Geometry check sheet. Reference: the model listing, model coordinates, mm. A direction names the side the tool comes from. Round coordinates to 2 decimals unless told otherwise and drop trailing zeros. Order: outer loops, then holes, each group sorted by start corner. A loop starts at its lowest first (then second) coordinate and runs counter-clockwise, first axis right, second up. Notation, with made-up numbers: M 13.25,32 L 37.25,32 A28 ccw 37.25,58 Z; hole C -2.5,-11.75 d11. An arc over 180 degrees is marked long. Return JSON: item names as keys, results as strings. Group by question number.
```python
from build123d import *

# Parameters (mm, degrees)
F1_DEPTH = 6.35


with BuildPart() as f1:
    # F0 (on Top) → F1 (new body)
    with BuildSketch(Plane.XY):
        with BuildLine():
            Line((1.27, 15.24), (-1.27, 15.24))
            ThreePointArc((-1.27, 15.24), (-2.121422, 13.939986), (-2.54, 12.443408))
            ThreePointArc((-2.54, 12.443408), (-3.578003, 12.185561), (-4.59063, 11.841289))
            ThreePointArc((-4.59063, 11.841289), (-5.751872, 12.87399), (-7.170974, 13.507318))
            Line((-7.170974, 13.507318), (-9.307758, 12.13409))
            ThreePointArc((-9.307758, 12.13409), (-9.321179, 10.580136), (-8.864198, 9.094833))
            ThreePointArc((-8.864198, 9.094833), (-9.59802, 8.316731), (-10.263768, 7.479644))
            ThreePointArc((-10.263768, 7.479644), (-11.798987, 7.720592), (-13.335215, 7.486157))
            Line((-13.335215, 7.486157), (-14.390369, 5.175692))
            ThreePointArc((-14.390369, 5.175692), (-13.561528, 3.861167), (-12.374076, 2.858713))
            ThreePointArc((-12.374076, 2.858713), (-12.570732, 1.807398), (-12.678232, 0.743265))
            ThreePointArc((-12.678232, 0.743265), (-14.100007, 0.115962), (-15.265619, -0.911805))
            Line((-15.265619, -0.911805), (-14.904139, -3.425951))
            ThreePointArc((-14.904139, -3.425951), (-13.496187, -4.083695), (-11.955272, -4.285028))
            ThreePointArc((-11.955272, -4.285028), (-11.552326, -5.275771), (-11.067446, -6.229095))
            ThreePointArc((-11.067446, -6.229095), (-11.924374, -7.525486), (-12.349297, -9.020276))
            Line((-12.349297, -9.020276), (-10.68595, -10.93988))
            ThreePointArc((-10.68595, -10.93988), (-9.145903, -10.732013), (-7.740754, -10.068303))
            ThreePointArc((-7.740754, -10.068303), (-6.866138, -10.68392), (-5.942825, -11.223762))
            ThreePointArc((-5.942825, -11.223762), (-5.962837, -12.777645), (-5.51216, -14.264873))
            Line((-5.51216, -14.264873), (-3.075048, -14.980473))
            ThreePointArc((-3.075048, -14.980473), (-1.891859, -13.972992), (-1.068601, -12.654963))
            ThreePointArc((-1.068601, -12.654963), (0, -12.7), (1.068601, -12.654963))
            ThreePointArc((1.068601, -12.654963), (1.891859, -13.972992), (3.075048, -14.980473))
            Line((3.075048, -14.980473), (5.51216, -14.264873))
            ThreePointArc((5.51216, -14.264873), (5.962837, -12.777645), (5.942825, -11.223762))
            ThreePointArc((5.942825, -11.223762), (6.866138, -10.68392), (7.740754, -10.068303))
            ThreePointArc((7.740754, -10.068303), (9.145903, -10.732013), (10.68595, -10.93988))
            Line((10.68595, -10.93988), (12.349297, -9.020276))
            ThreePointArc((12.349297, -9.020276), (11.924374, -7.525486), (11.067446, -6.229095))
            ThreePointArc((11.067446, -6.229095), (11.552326, -5.275771), (11.955272, -4.285028))
            ThreePointArc((11.955272, -4.285028), (13.496187, -4.083695), (14.904139, -3.425951))
            Line((14.904139, -3.425951), (15.265619, -0.911805))
            ThreePointArc((15.265619, -0.911805), (14.100007, 0.115962), (12.678232, 0.743265))
            ThreePointArc((12.678232, 0.743265), (12.570732, 1.807398), (12.374076, 2.858713))
            ThreePointArc((12.374076, 2.858713), (13.561528, 3.861167), (14.390369, 5.175692))
            Line((14.390369, 5.175692), (13.335215, 7.486157))
            ThreePointArc((13.335215, 7.486157), (11.798987, 7.720592), (10.263768, 7.479644))
            ThreePointArc((10.263768, 7.479644), (9.59802, 8.316731), (8.864198, 9.094833))
            ThreePointArc((8.864198, 9.094833), (9.321179, 10.580136), (9.307758, 12.13409))
            Line((9.307758, 12.13409), (7.170974, 13.507318))
            ThreePointArc((7.170974, 13.507318), (5.751872, 12.87399), (4.59063, 11.841289))
            ThreePointArc((4.59063, 11.841289), (3.578003, 12.185561), (2.54, 12.443408))
            ThreePointArc((2.54, 12.443408), (2.121422, 13.939986), (1.27, 15.24))
        make_face()
        with BuildLine():
            ThreePointArc((-1.717218, -6.1134), (0, 6.35), (1.717218, -6.1134))
            ThreePointArc((1.717218, -6.1134), (1.623593, -6.177189), (1.5875, -6.284575))
            Line((1.5875, -6.284575), (1.5875, -9.3472))
            ThreePointArc((1.5875, -9.3472), (1.535424, -9.472924), (1.4097, -9.525))
            Line((1.4097, -9.525), (-1.4097, -9.525))
            ThreePointArc((-1.4097, -9.525), (-1.535424, -9.472924), (-1.5875, -9.3472))
            Line((-1.5875, -9.3472), (-1.5875, -6.284575))
            ThreePointArc((-1.5875, -6.284575), (-1.623593, -6.177189), (-1.717218, -6.1134))
        make_face(mode=Mode.SUBTRACT)
    extrude(amount=F1_DEPTH)


solid = f1.part
```
Q1. Section check B-B on y = 0. Record the cut outline in (x, z).
Q2. Set-up check for faces 1 (the face through (-1.906, -13.989, 3.131)), 2 (the face through (-14.08, 0.13, 3.13)), 3 (the face through (13.547, 3.845, 3.131)), 4 (the face through (2.13, 13.92, 3.13)): record each of +Z, -Z, +X, -X, +Y, -Y from which the full face is reachable in a straight line by a thin tool's end or side.
Q3. Material ranges on line 1 along X through (y, z) = (11.5, 1.25); line 2 along X through (y, z) = (0, 5); line 3 along X through (y, z) = (3, 0.5), recorded low to high.
Q4. Section check A-A on x = 0. Record the cut outline in (y, z) (3 decimals).
Q5. Depth check by flat-ended pin: pin 1 Ø12 at (x, y) = (-4, 1.5) entering from +Z; pin 2 Ø0.9 at (y, z) = (-8.5, 4.5) entering from -X; pin 3 Ø2 at (x, z) = (-11.5, 4.5) entering from +Y; pin 4 Ø1.5 at (x, z) = (-3.5, 3.5) entering from +Y. Enter the tip coordinate at first touch or a pass-through.
Geometry check:
{
 "1": {"outline": "M -14.27,0 L -6.35,0 L -6.35,6.35 L -14.27,6.35 Z; M 6.35,0 L 14.27,0 L 14.27,6.35 L 6.35,6.35 Z"},
 "2": {"face 1": "+Z, -Z, -Y", "face 2": "+Z, -Z, -X", "face 3": "+Z, -Z, +X", "face 4": "+Z, -Z, +Y"},
 "3": {"line 1": "x = -9.37 to 9.37", "line 2": "x = -14.27 to -6.35, 6.35 to 14.27", "line 3": "x = -12.59 to -5.6, 5.6 to 12.59"},
 "4": {"outline": "M -12.7,0 L -9.525,0 L -9.525,6.35 L -12.7,6.35 Z; M 6.35,0 L 15.24,0 L 15.24,6.35 L 6.35,6.35 Z"},
 "5": {"pin 1": "stops at z = 6.35", "pin 2": "stops at x = -12.34", "pin 3": "stops at y = 7.72", "pin 4": "stops at y = 12.4"}
}
